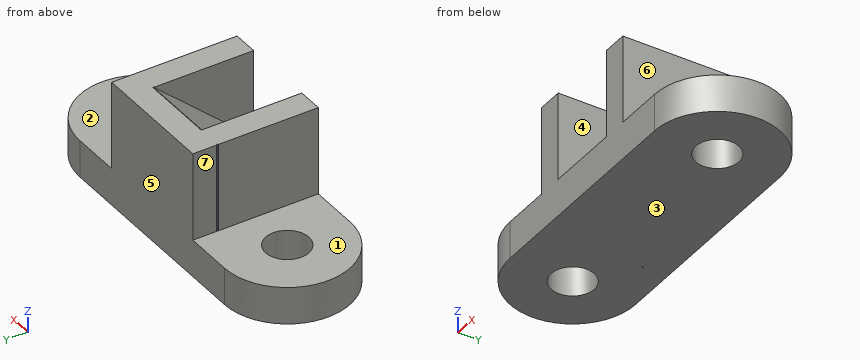
Autodesk Fusion 360 part; units mm, degrees
sketch "Sketch1" plane through (0, 0, 0) normal (0, 0, 1) x (1, 0, 0)
  line L0 (57, 32) -> (-57, 32)
  line L1 (-57, -32) -> (57, -32)
  circle A0 centre (57, 0) radius 11
  circle A1 centre (-57, 0) radius 11
  line L2 (-32, 32) -> (32, 32)
  line L3 (32, 32) -> (32, 19)
  line L4 (-32, 19) -> (-32, 32)
  arc A2 (-31.2512, 19) -> (-32, 19.975) centre (-57, 0) ccw
  arc A3 (-57, 32) -> (-57, -32) centre (-57, 0) ccw
  arc A4 (57, -32) -> (57, 32) centre (57, 0) ccw
  line L5 (-32, 19) -> (-31.2512, 19)
  line L6 (-19, 19) -> (-19, -32)
  line L7 (-19, -32) -> (-32, -32)
  line L8 (-32, -32) -> (-32, 19)
  line L9 (32, 19) -> (31.2512, 19)
  line L10 (19, 19) -> (19, -32)
  line L11 (19, -32) -> (32, -32)
  line L12 (32, -32) -> (32, 19)
  line L13 (-32, 17.9649) -> (-29.6806, 16.6628) construction
  line L14 (-31.2512, 19) -> (-32, 19)
  line L15 (32, 19) -> (31.2512, 19)
  line L16 (19, 19) -> (-19, 19)
  dimension "d1" = 114
  dimension "d2" = 64
  dimension "d3" = 22
  dimension "d4" = 22
  dimension "d5" = 64
  dimension "d6" = 13
  dimension "d8" = 13
  dimension "d9" = 13
extrude "Extrude1" add sketch "Sketch1" along normal blind 19 contours L0 L1 L3 A4 L12 makes body 1
extrude "Extrude2" add sketch "Sketch1" along normal blind 19 separate body contours L0 L1 L4 A3 L8 makes body 2
extrude "Extrude3" add sketch "Sketch1" along normal blind 19 separate body contours L1 L6 L10 L16 makes body 3
sketch "Sketch2" plane through (0, 0, 0) normal (1, 0, 0) x (0, 1, 0)
  line L0 (-31.7021, 19.3192) -> (19.2979, 19.3192)
  line L1 (19.2979, 19.3192) -> (19.2979, 64.3192)
  line L2 (19.2979, 64.3192) -> (-31.7021, 19.3192)
  dimension "d16" = 51
  dimension "d17" = 45
extrude "Extrude4" add sketch "Sketch1" along normal blind 64 contours L0 L1 L2 L3 L4 A2 L5 L6 L7 L8 L10 L11 L12 L14 L16 bodies 1 2 3
extrude "Extrude5" add sketch "Sketch2" along normal mid plane 38 bodies 1
equation "d6 = 64 mm - 51 mm"
equation "d17 = 64 mm - 19 mm"
Model file for the job. Use its own axes, mm. Face numbers are marked on the shaded views. A direction names the side the tool comes from. Give positions to 0.01 mm unless a question says otherwise; leave off trailing zeros. Order: outer loops, then holes, each group sorted by start corner. A loop starts at its lowest first (then second) coordinate and runs counter-clockwise, first axis right, second up.
1) Saw through at C-C, the plane x = -9. Write the cut outline in (y, z).
2) Wall check: probe 1 along Y at (x, z) = (-57, 6.25); probe 2 along X at (y, z) = (-16.5, 44.5); probe 3 along X at (y, z) = (18, 39). Give the ranges that are in metal, low to high.
3) Saw through at B-B, the plane x = -64. Write the cut outline in (y, z), then the cut area to 3 significant figures.
4) Mould opens along X. For the marked faces 4, 5, 6 and 7 say: +X half, -X half, draft (parallel to the pull), parting line (faces both ways), or undercut.
5) Pin check, flat tips, straight feed: pin 1 (5 mm diameter, centred on y = -14, z = 45, fed in from -X); pin 2 (12 mm diameter, centred on x = -47.5, y = -9.5, fed in from +Z); pin 3 (11.5 mm diameter, centred on x = -4, y = -5, fed in from +Z). Stop position of each tip, or through.
6) Saw through at A-A, the plane y = 0. Write the cut outline in (x, z), then the cut area to 3 significant figures.
7) 3-axis set-ups, long thin cutter, end or side, ignore diameter. For the marked faces 1, 2 and 3: which of +Z, -Z, +X, -X, +Y, -Y reach the whole face in a straight line?
8) Saw through at D-D, the plane z = 56. Write the cut outline in (x, y) (3 decimals).
Computed:
1. outline: (-32, 0) - (32, 0) - (32, 64) - (19.3, 64) - (19.3, 64.32) - (-31.7, 19.32) - (19, 19.32) - (19, 19) - (-32, 19) - close
2. probe 1: y = -32 to -11, 11 to 32
2. probe 2: x = -32 to -19, 19 to 32
2. probe 3: x = -32 to 32
3. outline: (-31.22, 0) - (-8.49, 0) - (-8.49, 19) - (-31.22, 19) - close; (8.49, 0) - (31.22, 0) - (31.22, 19) - (8.49, 19) - close
3. area: 864 mm2
4. face 4: undercut
4. face 5: draft
4. face 6: +X half
4. face 7: -X half
5. pin 1: stops at x = -32
5. pin 2: stops at z = 19
5. pin 3: stops at z = 47.95
6. outline: (-89, 0) - (-68, 0) - (-68, 19) - (-89, 19) - close; (-46, 0) - (46, 0) - (46, 19) - (32, 19) - (32, 64) - (19, 64) - (19, 47.29) - (-19, 47.29) - (-19, 64) - (-32, 64) - (-32, 19) - (-46, 19) - close; (68, 0) - (89, 0) - (89, 19) - (68, 19) - close; hole (-19, 19) - (19, 19) - (19, 19.32) - (-19, 19.32) - close
6. area: 4,780 mm2
7. face 1: +Z, -X, +Y, -Y
7. face 2: +Z, +X, +Y, -Y
7. face 3: -Z, +X, -X, +Y, -Y
8. outline: (-32, -32) - (-19, -32) - (-19, 9.869) - (19, 9.869) - (19, -32) - (32, -32) - (32, 32) - (-32, 32) - (-32, 19.975) arc R32 cw to (-31.251, 19) - (-32, 19) - close
